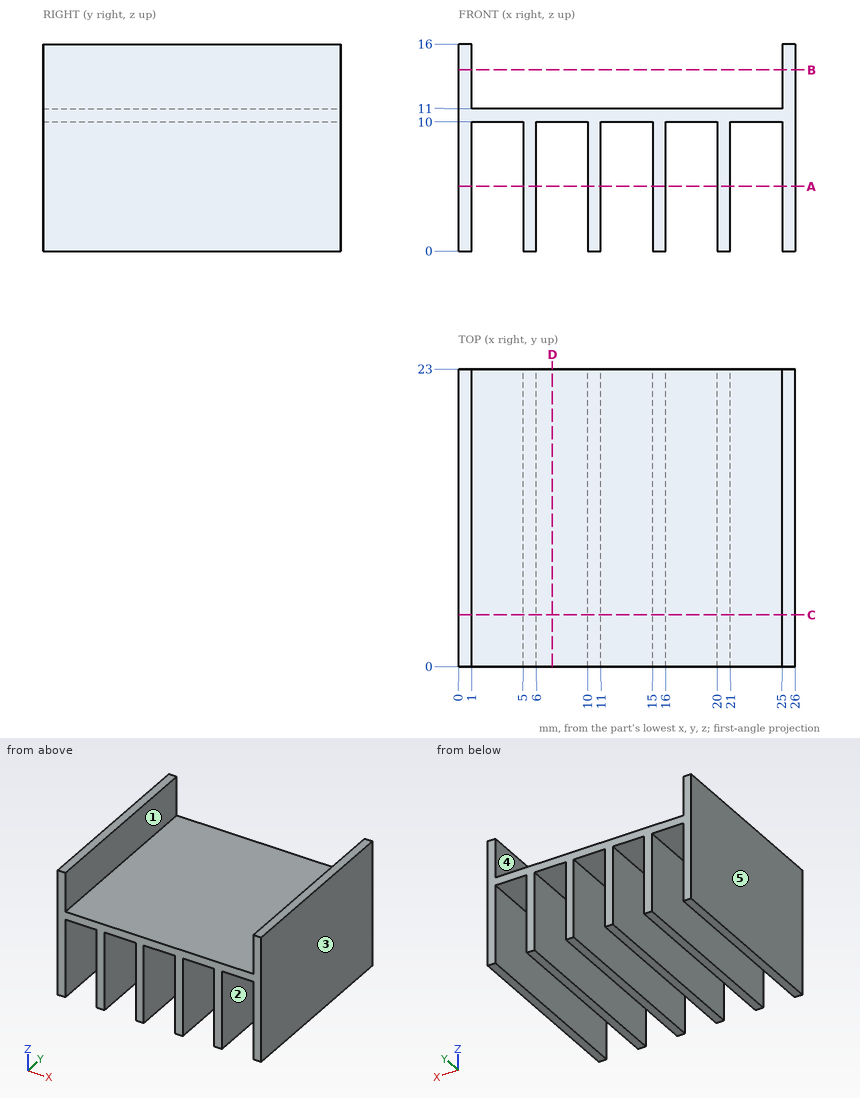
Could you check a few things on this drawing? It's one solid part, dimensions in mm from its lowest x, y, z. A direction names the side the tool comes from. Give positions to 0.01 mm unless a question says otherwise; leave off trailing zeros. Order: outer loops, then holes, each group sorted by start corner. A loop starts at its lowest first (then second) coordinate and runs counter-clockwise, first axis right, second up.
1. For pin 1 (1.2 mm diameter, centred on x = 4, y = 16, fed in from -Z); pin 2 (6 mm diameter, centred on x = 21.5, y = 15.5, fed in from +Z), each with a flat end and sliding along its axis, tell me the tip position at first contact or that it passes through.
Answers below:
pin 1: stops at z = 10
pin 2: stops at z = 11
2. Suppose I cut it at D-D (x = 7.25). Write out the boundary of the cut face in (y, z), plus the area to 3 significant figures.
Answers below:
outline: (0, 10) - (23, 10) - (23, 11) - (0, 11) - close
area: 23.0 mm2
3. I need wall thicknesses on L1, parallel to X at y = 10, z = 9; L2, parallel to X at y = 2.75, z = 14.5; L3, parallel to Z at x = 9.5, y = 21.5. Which ranges of each line are inside material? Lowest first, please.
Answers below:
L1: x = 0 to 1, 5 to 6, 10 to 11, 15 to 16, 20 to 21, 25 to 26
L2: x = 0 to 1, 25 to 26
L3: z = 10 to 11
4. Suppose I cut it at A-A (z = 5). Write out the boundary of the cut face in (x, y).
Answers below:
outline: (0, 0) - (1, 0) - (1, 23) - (0, 23) - close; (5, 0) - (6, 0) - (6, 23) - (5, 23) - close; (10, 0) - (11, 0) - (11, 23) - (10, 23) - close; (15, 0) - (16, 0) - (16, 23) - (15, 23) - close; (20, 0) - (21, 0) - (21, 23) - (20, 23) - close; (25, 0) - (26, 0) - (26, 23) - (25, 23) - close
5. Suppose I cut it at C-C (y = 4). Write out the boundary of the cut face in (x, z), plus the area to 3 significant figures.
Answers below:
outline: (0, 0) - (1, 0) - (1, 10) - (5, 10) - (5, 0) - (6, 0) - (6, 10) - (10, 10) - (10, 0) - (11, 0) - (11, 10) - (15, 10) - (15, 0) - (16, 0) - (16, 10) - (20, 10) - (20, 0) - (21, 0) - (21, 10) - (25, 10) - (25, 0) - (26, 0) - (26, 16) - (25, 16) - (25, 11) - (1, 11) - (1, 16) - (0, 16) - close
area: 96.0 mm2
6. Which directions (+Z, -Z, +X, -X, +Y, -Y) give clear straight access to the entire face, cutting with the end or side of a thin tool? Please do the marked faces 1 and 2.
Answers below:
face 1: +Z, +Y, -Y
face 2: -Z, +Y, -Y
7. Thinking about a two-plate mould opening in X: for the marked faces 3, 4 and 5, which applies, +X half, -X half, draft (parallel to the pull), parting line (faces both ways), or undercut?
Answers below:
face 3: +X half
face 4: undercut
face 5: -X half
8. Suppose I cut it at B-B (z = 14). Write out the boundary of the cut face in (x, y), plus the area to 3 significant figures.
Answers below:
outline: (0, 0) - (1, 0) - (1, 23) - (0, 23) - close; (25, 0) - (26, 0) - (26, 23) - (25, 23) - close
area: 46.0 mm2
